```python
from build123d import *

# Parameters (mm, degrees)
F2_R     = 1
F4_DEPTH = 27
F5_DEPTH = 27
F6_DEPTH = 15
F7_DEPTH = 15
F8_DEPTH = 15
F9_R     = 0.2


with BuildPart() as f1:
    # F0 (on Front) → F1 (revolve)
    with BuildSketch(Plane.XZ):
        Polygon((-9.0454753935, 4.269), (-9.0454753935, 2.769), (17.9545246065, 2.769), (17.9545246065, 3.769), (13.9545246065, 3.769), (13.9545246065, 4.269), (11.4545246065, 4.269), (10.9545246065, 4.569), (10.4545246065, 4.269), (7.9545246065, 4.269), (7.9545246065, 6.269), (5.9545246065, 6.269), (5.9545246065, 4.269), align=None)
    revolve(axis=Axis((2.1683473801, 0, 0), (1, 0, 0)))

    # F2
    f2_edges = [f1.edges().sort_by_distance(p)[0] for p in [
        (5.954525, 0, -6.269),
    ]]
    fillet(f2_edges, radius=F2_R)

    # F3 (on face) → F4 (join)
    with BuildSketch(Plane(origin=(-9.0454753935, 0, 0), x_dir=(0, -1, 0), z_dir=(-1, 0, 0))):
        with BuildLine():
            ThreePointArc((2.769, 0), (2.674648613, 0.7166699359), (2.3980243431, 1.3845))
            Line((2.3980243431, 1.3845), (2.3980243431, -1.3845))
            ThreePointArc((2.3980243431, -1.3845), (2.674648613, -0.7166699359), (2.769, 0))
        make_face()
    extrude(amount=-F4_DEPTH)

    # F3 (on face) → F5 (join)
    with BuildSketch(Plane(origin=(-9.0454753935, 0, 0), x_dir=(0, -1, 0), z_dir=(-1, 0, 0))):
        with BuildLine():
            ThreePointArc((2.769, 0), (2.674648613, 0.7166699359), (2.3980243431, 1.3845))
            Line((2.3980243431, 1.3845), (2.3980243431, -1.3845))
            ThreePointArc((2.3980243431, -1.3845), (2.674648613, -0.7166699359), (2.769, 0))
        make_face()
        with BuildLine():
            Line((1.921710371, 1.6595), (2.3980243431, 1.3845))
            ThreePointArc((2.3980243431, 1.3845), (2.2336171897, 1.6365559111), (2.0428279989, 1.8692818853))
            Line((2.0428279989, 1.8692818853), (1.921710371, 1.6595))
        make_face()
        with BuildLine():
            ThreePointArc((0.9910607425, -2.5855675595), (1.7978084575, -2.1060023148), (2.3980243431, -1.3845))
            Line((2.3980243431, -1.3845), (0.8227241336, -2.294))
            Line((0.8227241336, -2.294), (0.9910607425, -2.5855675595))
        make_face()
        with BuildLine():
            Line((0, 2.769), (1.5753002095, 1.8595))
            Line((1.5753002095, 1.8595), (1.7436368184, 2.1510675595))
            ThreePointArc((1.7436368184, 2.1510675595), (0.9249472763, 2.6099489528), (0, 2.769))
        make_face()
        with BuildLine():
            Line((0.5974316, -2.7037818853), (0.4763139721, -2.494))
            Line((0.4763139721, -2.494), (0, -2.769))
            ThreePointArc((0, -2.769), (0.3004903988, -2.7526471841), (0.5974316, -2.7037818853))
        make_face()
        with BuildLine():
            Line((-2.3980243431, 1.3845), (0, 2.769))
            ThreePointArc((0, 2.769), (-1.3845, 2.3980243431), (-2.3980243431, 1.3845))
        make_face()
        with BuildLine():
            ThreePointArc((-2.3980243431, -1.3845), (-1.3845, -2.3980243431), (0, -2.769))
            Line((0, -2.769), (-2.3980243431, -1.3845))
        make_face()
        with BuildLine():
            Line((-2.3980243431, 0.8345), (-2.3980243431, 1.3845))
            ThreePointArc((-2.3980243431, 1.3845), (-2.5341075885, 1.1160912731), (-2.640259599, 0.8345))
            Line((-2.640259599, 0.8345), (-2.3980243431, 0.8345))
        make_face()
        with BuildLine():
            ThreePointArc((-2.734697561, 0.4345), (-2.7227557338, -0.503946638), (-2.3980243431, -1.3845))
            Line((-2.3980243431, -1.3845), (-2.3980243431, 0.4345))
            Line((-2.3980243431, 0.4345), (-2.734697561, 0.4345))
        make_face()
    extrude(amount=-F5_DEPTH)

    # F3 (on face) → F6 (cut)
    with BuildSketch(Plane(origin=(-9.0454753935, 0, 0), x_dir=(0, -1, 0), z_dir=(-1, 0, 0))):
        with BuildLine():
            ThreePointArc((1.7436368184, 2.1510675595), (1.8984677361, 2.0157334286), (2.0428279989, 1.8692818853))
            Line((2.0428279989, 1.8692818853), (2.8160191704, 3.2084882783))
            ThreePointArc((2.8160191704, 3.2084882783), (2.6608491673, 3.3382993738), (2.4997033736, 3.4606132468))
            Line((2.4997033736, 3.4606132468), (1.7436368184, 2.1510675595))
        make_face()
    extrude(amount=-F6_DEPTH, mode=Mode.SUBTRACT)

    # F3 (on face) → F7 (cut)
    with BuildSketch(Plane(origin=(-9.0454753935, 0, 0), x_dir=(0, -1, 0), z_dir=(-1, 0, 0))):
        with BuildLine():
            Line((1.7471272977, -3.8951132468), (0.9910607425, -2.5855675595))
            ThreePointArc((0.9910607425, -2.5855675595), (0.7964424884, -2.651988002), (0.5974316, -2.7037818853))
            Line((0.5974316, -2.7037818853), (1.3706227715, -4.0429882783))
            ThreePointArc((1.3706227715, -4.0429882783), (1.5606274795, -3.9735126614), (1.7471272977, -3.8951132468))
        make_face()
    extrude(amount=-F7_DEPTH, mode=Mode.SUBTRACT)

    # F3 (on face) → F8 (cut)
    with BuildSketch(Plane(origin=(-9.0454753935, 0, 0), x_dir=(0, -1, 0), z_dir=(-1, 0, 0))):
        with BuildLine():
            Line((-2.640259599, 0.8345), (-4.1866419419, 0.8345))
            ThreePointArc((-4.1866419419, 0.8345), (-4.2214766468, 0.6352132876), (-4.2468306712, 0.4345))
            Line((-4.2468306712, 0.4345), (-2.734697561, 0.4345))
            ThreePointArc((-2.734697561, 0.4345), (-2.6949102244, 0.6362545734), (-2.640259599, 0.8345))
        make_face()
    extrude(amount=-F8_DEPTH, mode=Mode.SUBTRACT)

    # F9
    f9_edges = [f1.edges().sort_by_distance(p)[0] for p in [
        (-9.045475, 1.560627, 3.973513),
        (-9.045475, -4.221477, -0.635213),
        (-9.045475, 2.660849, -3.338299),
        (-9.045475, 2.398024, -0.475),
        (-9.045475, 1.199012, -2.07675),
        (-9.045475, -0.238157, -2.6315),
        (-9.045475, -2.398024, 0),
        (-9.045475, -2.159867, 1.522),
        (-9.045475, 1.199012, 2.07675),
        (-9.045475, -0.78765, 2.31425),
        (-9.045475, -1.610374, -1.83925),
        (-9.045475, 2.398024, 1.1095),
    ]]
    fillet(f9_edges, radius=F9_R)


solid = f1.part
```
Work out the finished part from the listing and answer in its coordinate system (mm). A direction names the side the tool comes from. Coordinates: 2 decimals unless noted, no trailing zeros. Loops run counter-clockwise (first coordinate to the right, second up) from the corner with the lowest first, then second, coordinate; pieces in that order, holes last.
1) Flat-ended cylindrical pins translate along their axes: pin 1 (2 mm diameter, centred on x = 10, z = -2.5, fed in from -Y); pin 2 (5 mm diameter, centred on x = 8, z = 3.5, fed in from +Y); pin 3 (3 mm diameter, centred on x = 10, z = -1.5, fed in from +Y). Find the tip coordinate at first contact, or state that the pin passes through.
Results:
pin 1: stops at y = -4.05
pin 2: stops at y = 6.19
pin 3: stops at y = 4.56
2) Section A-A (x = 2.5) is taken. Give the vertices of the cut face in (y, z), plus the area to 3 significant figures.
Results:
outline: (-2.82, 3.21) arc R4.27 ccw to (-1.75, -3.9) - (-0.82, -2.29) - (-2.4, -1.38) - (-2.4, 1.38) - (-1.92, 1.66) - close; (-2.5, 3.46) - (-1.58, 1.86) - (0, 2.77) - (2.4, 1.38) - (2.4, 0.83) - (4.19, 0.83) arc R4.27 ccw to start; (-1.37, -4.04) arc R4.27 ccw to (4.25, 0.43) - (2.4, 0.43) - (2.4, -1.38) - (0, -2.77) - (-0.48, -2.49) - close
area: 35.1 mm2
3) For faces 1 (the cylindrical face through (-1.55, 1.62, 3.95)), 2 (the flat face through (13.955, 4, 0)), 3 (the cylindrical face through (-8.99, 1.21, 2.14)), 4 (the flat face through (4.367, 1.216, 2.067)), 5 (the flat face through (7.955, 4, -3)), determine the directions among +Z, -Z, +X, -X, +Y, -Y from which every point of the face is accessible in a straight line to the end or side of a thin tool.
Results:
face 1: +Z, -X
face 2: +X
face 3: -X
face 4: +X, -X
face 5: none
4) For a pull along Z with two mould halves and no side action, classify faces 6 (the cylindrical face through (15.93, 3.68, -0.82)), 7 (the flat face through (-9.045, 2.2, -2.2)), 8 (the flat face through (4.37, 1.18, -2.09)) as +Z half, -Z half, draft (parallel to the pull), parting line (faces both ways), or undercut.
Results:
face 6: parting line
face 7: draft
face 8: undercut
5) Consider probe 1 along Y at (x, z) = (-6.75, 2.25); probe 2 along Y at (x, z) = (-1.25, 0); probe 3 along Y at (x, z) = (0, 2). Determine where each line is inside the solid, lowest interval first.
Results:
probe 1: y = -3.63 to -2.26, -1.8 to -0.9, 0.9 to 3.63
probe 2: y = -4.27 to -2.4, 2.4 to 4.27
probe 3: y = -3.77 to -2.12, -1.66 to -1.33, 1.33 to 3.77
